Geometry check sheet. Reference: the model listing, model coordinates, mm. A direction names the side the tool comes from. Coordinates: 2 decimals unless noted, no trailing zeros. Write each loop counter-clockwise with the first axis right and the second up, starting at its lowest first coordinate (ties: lowest second). Pieces come first, ordered by that corner, then holes. Notation, with made-up numbers: (51, 17) -> (90, 17) arc R25 ccw to (90, 46) -> close; hole circle Ø5 at (-25, 70.5). An arc over 180 degrees is marked (long way). Answer in a Markdown table with one row per item. Add a question column.
1. Depth check by flat-ended pin: P1, Ø1, axis at y = -1.5, z = 2.5, coming from the +X side; P2, Ø9, axis at x = 0.5, y = -3.5, coming from the +Z side; P3, Ø8, axis at y = -9.5, z = -1, coming from the +X side. Enter the tip coordinate at first touch or a pass-through.
2. Set-up check for faces 1 (the cylindrical face through (12.932, -5.362, 8.211)), 2 (the cylindrical face through (-2.17, -9.76, 0.1)), 3 (the cylindrical face through (8.394, 2.643, 0.915)): record each of +Z, -Z, +X, -X, +Y, -Y from which the full face is reachable in a straight line by a thin tool's end or side.
3. Cross-section at A-A on z = -6.5. Record the cut outline in (x, y), and give its area (3 significant figures).
4. Cross-section at D-D on z = 1.5. Record the cut outline in (x, y).
5. Cross-section at C-C on y = 8. Record the cut outline in (x, z).
6. Mould release check, pull along X, two halves, no side actions. Record for faces 4 (the cylindrical face through (-4.84, 11.15, 8.19)), 5 (the flat face through (3, 10, -7.4)), 6 (the cylindrical face through (3.434, 1.081, -3.344)), 7 (the cylindrical face through (12.932, 5.362, -8.211)): pulls with the +X half, pulls with the -X half, needs draft (parallel to the pull), parting line crosses it, or undercut.
7. Scan lines: L1, parallel to Z at x = -9.5, y = 10.25; L2, parallel to Y at x = 5.75, z = 8.55; L3, parallel to Y at x = -1, z = -0.5. Record each from-to range of solid material in increasing order. Write a range as from..to.
8. Cross-section at B-B on x = 5.75. Record the cut outline in (y, z), and give its area (3 significant figures).
Autodesk Inventor part; units mm, degrees
ref_plane "YZ Plane" through (0, 0, 0) normal (1, 0, 0) x (0, 1, 0)
ref_plane "XZ Plane" through (0, 0, 0) normal (0, 1, 0) x (-1, 0, 0)
ref_plane "XY Plane" through (0, 0, 0) normal (0, 0, 1) x (1, 0, 0)
sketch "Sketch1" plane through (0, 0, 0) normal (0, 0, 1) x (1, 0, 0)
  circle A0 centre (0, 0) radius 10
  dimension "d0" = 20
extrude "Extrusion1" add sketch "Sketch1" along normal mid plane 18
sketch "Sketch2" plane through (0, 0, -9) normal (0, 0, -1) x (-1, 0, 0)
  point P0 (0, 0)
hole "Hole1" at (0, 0, -9) direction (0, 0, 1) diameter 3.2 end through all
sketch "Sketch3" plane through (0, 0, 9) normal (0, 0, 1) x (1, 0, 0)
  circle A0 centre (0, 0) radius 14
  circle A1 centre (0, 0) radius 10
  dimension "d10" = 28
extrude "Extrusion2" add sketch "Sketch3" against normal blind 1.6
mirror "Mirror1" about plane through (0, 0, 0) normal (0, 0, 1) of "Extrusion2"
sketch "Sketch4" plane through (0, 0, 9) normal (0, 0, 1) x (1, 0, 0)
  circle A0 centre (0, 0) radius 10
  circle A1 centre (0, 0) radius 10
  circle A2 centre (0, 0) radius 1.6
  circle A3 centre (0, 0) radius 8.8
  circle A4 centre (0, 0) radius 3.6
  dimension "d13" = 1.2
  dimension "d14" = 2
extrude "Extrusion3" cut sketch "Sketch4" against normal up to surface (16.4 mm away) contours A3
sketch "Sketch5" plane through (0, 0, 9) normal (0, 0, 1) x (1, 0, 0)
  circle A0 centre (0, 0) radius 3.6
extrude "Extrusion4" cut sketch "Sketch5" against normal blind 8.4
sketch "Sketch8" plane through (0, 0, 7.4) normal (0, 0, 1) x (1, 0, 0)
  line L0 (0, -19.6) -> (0, 19.6)
  circle A0 centre (0, 0) radius 10
  circle A1 centre (0, 11.5) radius 1.5
  dimension "d36" = 3
extrude "Extrusion6" cut sketch "Sketch8" along normal through all contours A1 L0 | L0 A1
pattern_circular "Circular Pattern1" count 12 over 360 about axis through (0, 0, -10) along (0, 0, 1) of "Extrusion6"
properties part number "SpoolTraditionalMachining"
Results found:
| question | item | result |
|---|---|---|
| 1 | P1 | stops at x = 9.95 |
| 1 | P2 | stops at z = 0.6 |
| 1 | P3 | stops at x = 8.35 |
| 2 | face 1 | +Z, -Z |
| 2 | face 2 | none |
| 2 | face 3 | +Z |
| 3 | outline | circle Ø20 at (0, 0); circle Ø7.2 at (0, 0); hole circle Ø17.6 at (0, 0); hole circle Ø3.2 at (0, 0) |
| 3 | area | 104 mm^2 |
| 4 | outline | circle Ø20 at (0, 0); hole circle Ø17.6 at (0, 0) |
| 5 | outline | (-11.49, -9) -> (11.49, -9) -> (11.49, -7.4) -> (6, -7.4) -> (6, 7.4) -> (11.49, 7.4) -> (11.49, 9) -> (3.67, 9) -> (3.67, -7.4) -> (-3.67, -7.4) -> (-3.67, 9) -> (-11.49, 9) -> (-11.49, 7.4) -> (-6, 7.4) -> (-6, -7.4) -> (-11.49, -7.4) -> close |
| 6 | face 4 | undercut |
| 6 | face 5 | needs draft |
| 6 | face 6 | undercut |
| 6 | face 7 | parting line crosses it |
| 7 | L1 | z = -9..-7.4, 7.4..9 |
| 7 | L2 | y = -12.76..-11.46, -8.46..-6.66, 6.66..8.46, 11.46..12.76 |
| 7 | L3 | y = -9.95..-8.74, -3.46..-1.25, 1.25..3.46, 8.74..9.95 |
| 8 | outline | (-12.76, -9) -> (12.76, -9) -> (12.76, -7.4) -> (8.18, -7.4) -> (8.18, 7.4) -> (8.46, 7.4) -> (8.46, 9) -> (6.66, 9) -> (6.66, -7.4) -> (-6.66, -7.4) -> (-6.66, 9) -> (-8.46, 9) -> (-8.46, 7.4) -> (-8.18, 7.4) -> (-8.18, -7.4) -> (-12.76, -7.4) -> close; (-12.76, 7.4) -> (-11.46, 7.4) -> (-11.46, 9) -> (-12.76, 9) -> close; (11.46, 7.4) -> (12.76, 7.4) -> (12.76, 9) -> (11.46, 9) -> close |
| 8 | area | 95.8 mm^2 |
